```python
from build123d import *

# Parameters (mm, degrees)
F0_W     = 62.2431822121
F0_H     = 47.7795563638
F1_DEPTH = 34.29
F2_SIZE  = 5.08
F4_D     = 10


with BuildPart() as f1:
    # F0 (on Top) → F1 (new body)
    with BuildSketch(Plane.XY):
        with Locations((-85.0962679833, -23.8897781819)):
            Rectangle(F0_W, F0_H)
    extrude(amount=F1_DEPTH)

    # F2
    f2_edges = [f1.edges().sort_by_distance(p)[0] for p in [
        (-116.217859, -47.779556, 17.145),
        (-53.974677, -47.779556, 17.145),
        (-85.096268, -47.779556, 0),
        (-85.096268, -47.779556, 34.29),
        (-85.096268, 0, 34.29),
        (-116.217859, -23.889778, 34.29),
        (-53.974677, -23.889778, 34.29),
        (-53.974677, 0, 17.145),
        (-53.974677, -23.889778, 0),
        (-116.217859, 0, 17.145),
        (-116.217859, -23.889778, 0),
        (-85.096268, 0, 0),
    ]]
    chamfer(f2_edges, length=F2_SIZE)

    # F4 (through all)
    with Locations(Plane.XY.offset(34.29)):
        with Locations((-86.2206369638, -19.9478901923)):
            Hole(F4_D / 2)


solid = f1.part
```
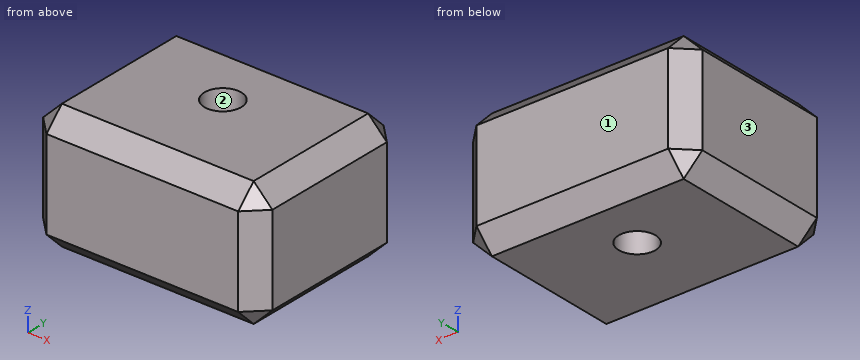
For this review, take the finished solid that the model builds, in its own axes (mm). Face numbers are marked on the shaded views. Give positions to 0.01 mm unless a question says otherwise; leave off trailing zeros. Write each loop counter-clockwise with the first axis right and the second up, starting at its lowest first coordinate (ties: lowest second). Pieces come first, ordered by that corner, then holes. Notation, with made-up numbers: M 87,59 L 139,59 A9 cw 139,74 Z; hole C 11,63 d7. An arc over 180 degrees is marked long. Answer as a JSON object with one key per item and string values. Group by question number.
Item 1: Consider section A-A on x = -71.5. Write out the cut boundary in (y, z).
Item 2: Consider section C-C on x = -87. Write out the cut boundary in (y, z).
Item 3: For pin 1 Ø8 at (x, z) = (-83.5, 29.5) entering from +Y; pin 2 Ø9 at (x, y) = (-86.22, -19.95) entering from +Z, all flat-tipped, find the tip position at first contact; note any pin that passes through.
Item 4: Consider section D-D on y = -41. Write out the cut boundary in (x, z).
Item 5: Draft analysis for pull direction Y (two halves, no side actions). For the marked faces 1, 2 and 3, state which applies: +Y half, -Y half, draft (parallel to the pull), parting line (faces both ways), or undercut.
Item 6: For probe 1 along X at (y, z) = (-24, 26); probe 2 along X at (y, z) = (-18, 31.5); probe 3 along Y at (x, z) = (-90.5, 12), list the stretches that pass through material, from the lowest coordinate up. Write a range as [from, to].
Item 7: Consider section B-B on y = -16.5. Write out the cut boundary in (x, z), plus the area to 3 significant figures.
Check result:
{
 "1": {"outline": "M -47.78,5.08 L -42.7,0 L -5.08,0 L 0,5.08 L 0,29.21 L -5.08,34.29 L -42.7,34.29 L -47.78,29.21 Z"},
 "2": {"outline": "M -47.78,5.08 L -42.7,0 L -24.89,0 L -24.89,34.29 L -42.7,34.29 L -47.78,29.21 Z; M -15.01,0 L -5.08,0 L 0,5.08 L 0,29.21 L -5.08,34.29 L -15.01,34.29 Z"},
 "3": {"pin 1": "stops at y = 0", "pin 2": "passes through"},
 "4": {"outline": "M -116.22,5.08 L -111.14,0 L -59.05,0 L -53.97,5.08 L -53.97,29.21 L -59.05,34.29 L -111.14,34.29 L -116.22,29.21 Z"},
 "5": {"face 1": "+Y half", "face 2": "undercut", "face 3": "draft"},
 "6": {"probe 1": "x = [-116.22, -89.15], [-83.29, -53.97]", "probe 2": "x = [-113.93, -90.83], [-81.62, -56.26]", "probe 3": "y = [-47.78, -22.53], [-17.36, 0]"},
 "7": {"outline": "M -116.22,5.08 L -111.14,0 L -89.84,0 L -89.84,34.29 L -111.14,34.29 L -116.22,29.21 Z; M -82.6,0 L -59.05,0 L -53.97,5.08 L -53.97,29.21 L -59.05,34.29 L -82.6,34.29 Z", "area": "1,830 mm^2"}
}
